Autodesk Inventor part; units mm, degrees
ref_plane "YZ Plane" through (0, 0, 0) normal (1, 0, 0) x (0, 1, 0)
ref_plane "XZ Plane" through (0, 0, 0) normal (0, 1, 0) x (-1, 0, 0)
ref_plane "XY Plane" through (0, 0, 0) normal (0, 0, 1) x (1, 0, 0)
sketch "Esquisse1" plane through (0, 0, 0) normal (0, 1, 0) x (-1, 0, 0)
  line L0 (-25, 15) -> (25, 15)
  line L1 (25, 15) -> (25, -15)
  line L2 (25, -15) -> (-25, -15)
  line L3 (-25, -15) -> (-25, 15)
  line L4 (-25, 15) -> (25, -15) construction
  line L5 (25, 15) -> (-25, -15) construction
  line L6 (-22, 12) -> (22, 12)
  line L7 (22, 12) -> (22, -12)
  line L8 (22, -12) -> (-22, -12)
  line L9 (-22, -12) -> (-22, 12)
  line L10 (-22, 12) -> (22, -12) construction
  line L11 (22, 12) -> (-22, -12) construction
  point P0 (0, 0)
  dimension "d0" = 50
  dimension "d1" = 30
  dimension "d2" = 3
  dimension "d3" = 3
extrude "Extrusion1" add sketch "Esquisse1" along normal blind 5 contours L0 L1 L2 L3 | L6 L7 L8 L9
sketch "Esquisse2" plane through (0, 0, 0) normal (0, -1, 0) x (1, 0, 0)
  line L0 (-22, 12) -> (22, 12)
  line L1 (22, 12) -> (22, -12)
  line L2 (22, -12) -> (-22, -12)
  line L3 (-22, -12) -> (-22, 12)
  line L4 (-22, 12) -> (22, -12) construction
  line L5 (22, 12) -> (-22, -12) construction
  line L6 (-25, -15) -> (25, -15)
  line L7 (25, -15) -> (25, 15)
  line L8 (25, 15) -> (-25, 15)
  line L9 (-25, 15) -> (-25, -15)
  point P0 (0, 0)
  dimension "d6" = 3
  dimension "d7" = 3
extrude "Extrusion2" add sketch "Esquisse2" along normal blind 60
sketch "Esquisse3" plane through (0, -60, 0) normal (0, -1, 0) x (1, 0, 0)
  line L0 (25, -15) -> (25, 15)
  line L1 (-25, -15) -> (25, -15)
  line L2 (25, 15) -> (-25, 15)
  line L3 (-25, 15) -> (-25, -15)
  point P0 (0, 0)
extrude "Extrusion3" add sketch "Esquisse3" along normal blind 5
sketch "Esquisse4" plane through (0, 5, 0) normal (0, 1, 0) x (1, 0, 0)
  point P0 (0, 0)
properties part number "Pièce_roue folle"
The listing builds one solid part. Answer for the finished solid, in the listing's coordinates (mm). A direction names the side the tool comes from. Coordinates: 2 decimals unless noted, no trailing zeros. Write each loop counter-clockwise with the first axis right and the second up, starting at its lowest first coordinate (ties: lowest second). Pieces come first, ordered by that corner, then holes. Notation, with made-up numbers: (43, 22) - (73, 22) arc R26 cw to (73, 43) - close; hole circle Ø2 at (37, 89). An arc over 180 degrees is marked (long way). Return JSON: item names as keys, results as strings. Group by question number.
1. A cutting plane is placed at B-B, the plane z = 10.5. Determine the outline of the cut face in (x, y), plus the area to 3 significant figures.
2. A cutting plane is placed at A-A, the plane y = -32.5. Determine the outline of the cut face in (x, z), plus the area to 3 significant figures.
3. Which of the six approach directions +Z, -Z, +X, -X, +Y, -Y give full straight-line access (tool end or side, diameter ignored) to faces 1 (the flat face through (0, -60, 0)), 2 (the flat face through (0, -30, 15))?
4. Straight lines are drawn through the part: L1, parallel to Y at x = 3.5, z = -1.75; L2, parallel to Z at x = -9.5, y = -24; L3, parallel to X at y = -35.5, z = -5.75. For each, find the intervals that lie inside material, in ascending order.
5. Determine the mould class of faces 3 (the flat face through (25, -30, 0)), 4 (the flat face through (22, -30, 0)), 5 (the flat face through (0, 5, 0)) for opening direction Y: released by +Y, released by -Y, zero draft, split by the parting line, or undercut.
Ans:
{
 "1": {"outline": "(-25, -65) - (25, -65) - (25, 5) - (-25, 5) - close; hole (-22, -60) - (22, -60) - (22, 0) - (-22, 0) - close", "area": "860 mm²"},
 "2": {"outline": "(-25, -15) - (25, -15) - (25, 15) - (-25, 15) - close; hole (-22, -12) - (22, -12) - (22, 12) - (-22, 12) - close", "area": "444 mm²"},
 "3": {"face 1": "none", "face 2": "+Z, +X, -X, +Y, -Y"},
 "4": {"L1": "-65 to -60, 0 to 5", "L2": "-15 to -12, 12 to 15", "L3": "-25 to -22, 22 to 25"},
 "5": {"face 3": "zero draft", "face 4": "undercut", "face 5": "released by +Y"}
}
